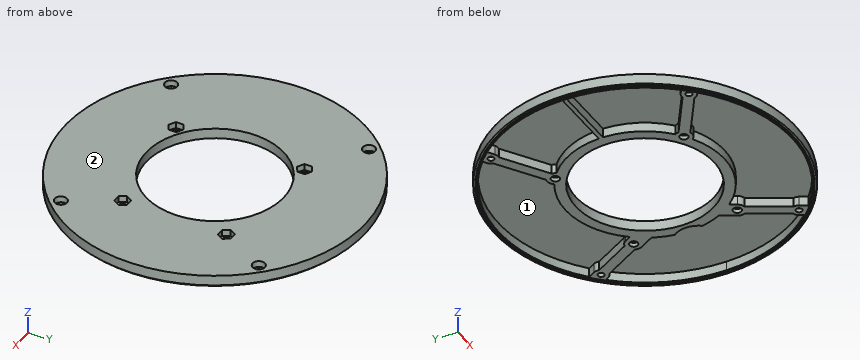
from build123d import *

# Parameters (mm, degrees)
SKIZZE1_R                 = 72.5
SKIZZE1_R_2               = 33.25
LIDAR_TOP_BASE_DEPTH      = 5
LIDAR_SCREWS_D            = 4
SPACER_SCREWS_D           = 3
SPACER_SCREWS_CBORE_D     = 6
SPACER_SCREWS_CBORE_DEPTH = 3
BOTTOM_START              = -4.5
BOTTOM_STRUCTURE_DEPTH    = 4.5
HEX_NUT_DEPTH             = 3
SKIZZE7_R                 = 71.5
SKIZZE7_R_2               = 71
COVER_RING_DEPTH          = 1


with BuildPart() as part:
    # Skizze1 → Lidar Top Base (new body)
    with BuildSketch(Plane.XY):
        Circle(SKIZZE1_R)
        Circle(SKIZZE1_R_2, mode=Mode.SUBTRACT)
    extrude(amount=LIDAR_TOP_BASE_DEPTH)

    # Lidar Screws (through all)
    with Locations(Plane.XY.offset(5)):
        with Locations((-22, 31), (35, 25), (35, -25), (-22, -31)):
            Hole(LIDAR_SCREWS_D / 2)

    # Spacer Screws (through all)
    with Locations(Plane(origin=(0, 0, 5), x_dir=(-1, 0, 0), z_dir=(0, 0, 1))):
        with Locations((47.72970773, -47.72970773), (47.72970773, 47.72970773), (-47.72970773, 47.72970773), (-47.72970773, -47.72970773)):
            CounterBoreHole(SPACER_SCREWS_D / 2, SPACER_SCREWS_CBORE_D / 2, SPACER_SCREWS_CBORE_DEPTH)

    # Skizze6 → Bottom Structure (cut)
    with BuildSketch(Plane(origin=(0, 0, 0), x_dir=(-1, 0, 0), z_dir=(0, 0, -1)).offset(BOTTOM_START)):
        with BuildLine():
            ThreePointArc((-44.67599804, 49.439929098), (-44.256119002, 48.158871274), (-44.351580895, 46.814142832))
            Line((-44.351580895, 46.814142832), (-34.344540081, 28.945931106))
            ThreePointArc((-34.344540081, 28.945931106), (-32.700538124, 28.272991763), (-31.510046068, 26.954538706))
            Line((-31.510046068, 26.954538706), (-29.825905448, 23.947397859))
            ThreePointArc((-29.825905448, 23.947397859), (-7.258760505, 37.554931713), (18.753747138, 33.337058483))
            ThreePointArc((18.753747138, 33.337058483), (20.765145539, 34.804620146), (23.255008426, 34.798019728))
            Line((23.255008426, 34.798019728), (44.31336561, 48.490369623))
            ThreePointArc((44.31336561, 48.490369623), (44.854292699, 49.725199749), (45.821815788, 50.663979077))
            Line((45.821815788, 50.663979077), (47.717721333, 51.896715414))
            ThreePointArc((47.717721333, 51.896715414), (0.745045066, 70.496063066), (-46.61023353, 52.893630338))
            Line((-46.61023353, 52.893630338), (-44.67599804, 49.439929098))
        make_face()
        with BuildLine():
            Line((-38.706982496, 26.502757723), (-48.714023309, 44.370969449))
            ThreePointArc((-48.714023309, 44.370969449), (-49.910490622, 44.992156639), (-50.78341742, 46.019486362))
            Line((-50.78341742, 46.019486362), (-51.795828593, 47.827211296))
            ThreePointArc((-51.795828593, 47.827211296), (-65.657657268, 25.677267029), (-70.5, 0))
            Line((-70.5, 0), (-57.456439237, 0))
            ThreePointArc((-57.456439237, 0), (-42.965235741, -10.431275001), (-37.672530483, 6.621400682))
            ThreePointArc((-37.672530483, 6.621400682), (-36.478038354, 11.507181142), (-34.652808242, 16.193992125))
            Line((-34.652808242, 16.193992125), (-38.489953932, 23.045461294))
            ThreePointArc((-38.489953932, 23.045461294), (-38.992142049, 24.749397), (-38.706982496, 26.502757723))
        make_face()
        with BuildLine():
            ThreePointArc((49.637599672, 44.795436383), (48.387022114, 44.291984966), (47.038925526, 44.298553413))
            Line((47.038925526, 44.298553413), (25.980568343, 30.606203517))
            ThreePointArc((25.980568343, 30.606203517), (25.751268172, 29.611480247), (25.277654247, 28.707188922))
            ThreePointArc((25.277654247, 28.707188922), (34.647475396, 16.205398751), (38.23692587, 1))
            Line((38.23692587, 1), (70.492907445, 1))
            ThreePointArc((70.492907445, 1), (65.727115081, 25.498947882), (52.72387838, 46.802164998))
            Line((52.72387838, 46.802164998), (49.637599672, 44.795436383))
        make_face()
    bottom_structure = extrude(amount=BOTTOM_STRUCTURE_DEPTH, mode=Mode.SUBTRACT)

    # Skizze9 → Hex Nut (cut)
    with BuildSketch(Plane.XY.offset(5)):
        Polygon((-18.875, 32.804219591), (-22, 34.608439182), (-25.125, 32.804219591), (-25.125, 29.195780409), (-22, 27.391560818), (-18.875, 29.195780409), align=None)
        Polygon((38.608439182, 25), (36.804219591, 28.125), (33.195780409, 28.125), (31.391560818, 25), (33.195780409, 21.875), (36.804219591, 21.875), align=None)
    hex_nut = extrude(amount=-HEX_NUT_DEPTH, mode=Mode.SUBTRACT)

    # Structure Mirror: Bottom Structure, Hex Nut across plane
    add(bottom_structure.mirror(Plane.ZX), mode=Mode.SUBTRACT)
    add(hex_nut.mirror(Plane.ZX), mode=Mode.SUBTRACT)

    # Skizze7 → Cover Ring (add)
    with BuildSketch(Plane(origin=(0, 0, 0), x_dir=(-1, 0, 0), z_dir=(0, 0, -1))):
        with Locations(Location((0, 0, 0), (0, 0, 180))):
            Circle(SKIZZE7_R)
        Circle(SKIZZE7_R_2, mode=Mode.SUBTRACT)
    extrude(amount=COVER_RING_DEPTH)


solid = part.part
Check sheet for the modelled part. Datum: model origin and axes. Units: mm. Face numbers are marked on the shaded views. Give positions to 0.01 mm unless a question says otherwise; leave off trailing zeros. Loops run counter-clockwise (first coordinate to the right, second up) from the corner with the lowest first, then second, coordinate; pieces in that order, holes last. Notation, with made-up numbers: M 4.25,81.25 L 35.25,81.25 A25 ccw 35.25,96.25 Z; hole C 78,83 d7. An arc over 180 degrees is marked long. Answer as a JSON object with one key per item and string values. Group by question number.
Q1. Release check for a two-part mould opening along Y. For the marked faces 1 and 2 record: released by +Y, released by -Y, zero draft, split by the parting line, or undercut.
Q2. Cross-section at A-A on x = 24.5. Record the cut outline in (y, z).
Q3. Cross-section at D-D on x = 56. Record the cut outline in (y, z), then the cut area to 3 significant figures.
Q4. Go/stop test with flat-tipped pins: P1, Ø14, axis at x = -7, y = 53.5, coming from the -Z side; P2, Ø1.5, axis at x = 34.5, z = 4, coming from the +Y side; P3, Ø1.5, axis at y = -31.5, z = 4, coming from the -X side; P4, Ø6.5, axis at x = 48.5, y = -48.5, coming from the +Z side. Record where each tip stops, or that it passes through.
Q5. Cross-section at B-B on y = 58. Record the cut outline in (x, z).
Q6. Material ranges on line 1 along Y through (x, z) = (-54.5, 1.4); line 2 along Y through (x, z) = (0, -0.4); line 3 along Y through (x, z) = (-28.5, 3.65), recorded low to high. Write a range as [from, to].
Evaluation:
{
 "1": {"face 1": "undercut", "face 2": "zero draft"},
 "2": {"outline": "M -68.23,0 L -67.17,0 L -67.17,-1 L -66.64,-1 L -66.64,0 L -66.11,0 L -66.11,4.5 L -29.37,4.5 L -29.37,0 L -22.48,0 L -22.48,5 L -68.23,5 Z; M 22.48,0 L 29.37,0 L 29.37,4.5 L 66.11,4.5 L 66.11,0 L 66.64,0 L 66.64,-1 L 67.17,-1 L 67.17,0 L 68.23,0 L 68.23,5 L 22.48,5 Z"},
 "3": {"outline": "M -46.05,0 L -44.46,0 L -44.46,-1 L -43.65,-1 L -43.65,0 L -42.83,0 L -42.83,4.5 L 42.83,4.5 L 42.83,0 L 43.65,0 L 43.65,-1 L 44.46,-1 L 44.46,0 L 46.05,0 L 46.05,5 L -46.05,5 Z", "area": "76.6 mm2"},
 "4": {"P1": "stops at z = 4.5", "P2": "stops at y = 64.17", "P3": "stops at x = -65.66", "P4": "stops at z = 5"},
 "5": {"outline": "M -43.5,0 L -41.81,0 L -41.81,-1 L -40.95,-1 L -40.95,0 L -40.08,0 L -40.08,4.5 L 40.08,4.5 L 40.08,0 L 40.95,0 L 40.95,-1 L 41.81,-1 L 41.81,0 L 43.5,0 L 43.5,5 L -43.5,5 Z"},
 "6": {"line 1": "y = [-47.81, -44.72], [-1, 1], [44.72, 47.81]", "line 2": "y = [-71.5, -71], [71, 71.5]", "line 3": "y = [-66.66, -64.48], [-38.21, -32.24], [-25.51, -17.13], [17.13, 25.51], [32.24, 38.21], [64.48, 66.66]"}
}
